from build123d import *

# Parameters (mm, degrees)
SKETCH1_R           = 30
BOSS_EXTRUDE1_DEPTH = 10
SKETCH2_W           = 30
SKETCH2_H           = 30
BOSS_EXTRUDE2_DEPTH = 40
SKETCH3_R           = 4.196967066
BOSS_EXTRUDE3_DEPTH = 110


with BuildPart() as part:
    # Sketch1 → Boss-Extrude1 (new body)
    with BuildSketch(Plane(origin=(0, 0, 0), x_dir=(1, 0, 0), z_dir=(0, 1, 0))):
        Circle(SKETCH1_R)
    extrude(amount=BOSS_EXTRUDE1_DEPTH)

    # Sketch2 → Boss-Extrude2 (add)
    with BuildSketch(Plane(origin=(0, 10, 0), x_dir=(1, 0, 0), z_dir=(0, 1, 0))):
        Rectangle(SKETCH2_W, SKETCH2_H)
    extrude(amount=BOSS_EXTRUDE2_DEPTH)

    # Sketch3 → Boss-Extrude3 (add)
    with BuildSketch(Plane(origin=(0, 50, 0), x_dir=(1, 0, 0), z_dir=(0, 1, 0))):
        Circle(SKETCH3_R)
    extrude(amount=BOSS_EXTRUDE3_DEPTH)


solid = part.part
Verification items for the finished model (mm, model axes). A direction names the side the tool comes from. Coordinates: 2 decimals unless noted, no trailing zeros. Order: outer loops, then holes, each group sorted by start corner. A loop starts at its lowest first (then second) coordinate and runs counter-clockwise, first axis right, second up. Notation, with made-up numbers: M 34,40.25 L 82,40.25 A11 cw 82,50.25 Z; hole C -38.5,46.5 d5. An arc over 180 degrees is marked long. One line per item, written item: value. Start each with the question number.
Item 1: Sectioned sample at B-B (x = -9.5). Enter the section's corners in (y, z), then the cut area to 3 significant figures.
Item 2: Access from +Z, -Z, +X, -X, +Y, -Y to the whole of each face (thin tool, end or side, straight path). Record for faces 1 (the cylindrical face through (-3.331, 104.23, 2.554)), 2 (the flat face through (15, 30, 0)), 3 (the flat face through (-15, 30, 0)), 4 (the flat face through (0, 30, 15)), 5 (the flat face through (0, 30, -15)).
Item 3: Sectioned sample at A-A (z = 0). Enter the section's corners in (x, y), then the cut area to 3 significant figures.
Item 4: Scan lines: probe 1 along Y at (x, z) = (-23.5, 1.5); probe 2 along X at (y, z) = (26, -10.5). Record each from-to range of solid material in increasing order.
Item 5: Gauge pin test, flat ends, axial feed: pin 1 (1 mm diameter, centred on x = 10, y = 28.5, fed in from -Z); pin 2 (10 mm diameter, centred on x = 11.5, z = 17, fed in from +Y); pin 3 (9 mm diameter, centred on y = 36, z = 4, fed in from +X). Record the tip position at first contact, or that the pin passes through.
Item 6: Sectioned sample at D-D (x = 0). Enter the section's corners in (y, z).
Item 7: Sectioned sample at C-C (y = 86). Enter the section's corners in (x, z).
Conclusion:
1. outline: M 0,-28.46 L 10,-28.46 L 10,-15 L 50,-15 L 50,15 L 10,15 L 10,28.46 L 0,28.46 Z
1. area: 1,770 mm^2
2. face 1: +Y
2. face 2: +Z, -Z, +X, +Y
2. face 3: +Z, -Z, -X, +Y
2. face 4: +Z, +X, -X, +Y
2. face 5: -Z, +X, -X, +Y
3. outline: M -30,0 L 30,0 L 30,10 L 15,10 L 15,50 L 4.2,50 L 4.2,160 L -4.2,160 L -4.2,50 L -15,50 L -15,10 L -30,10 Z
3. area: 2,720 mm^2
4. probe 1: y = 0 to 10
4. probe 2: x = -15 to 15
5. pin 1: stops at z = -15
5. pin 2: stops at y = 50
5. pin 3: stops at x = 15
6. outline: M 0,-30 L 10,-30 L 10,-15 L 50,-15 L 50,-4.2 L 160,-4.2 L 160,4.2 L 50,4.2 L 50,15 L 10,15 L 10,30 L 0,30 Z
7. outline: C 0,0 d8.39
